Source: CAD feature listing. Evaluate the final solid. Frame: model axes, mm. A direction names the side the tool comes from. Round coordinates to 2 decimals unless told otherwise and drop trailing zeros. Loops run counter-clockwise (first coordinate to the right, second up) from the corner with the lowest first, then second, coordinate; pieces in that order, holes last. Notation, with made-up numbers: (-5.5, 79) - (32.5, 79) arc R16 cw to (32.5, 94) - close; hole circle Ø9 at (-39.5, 77.25). An arc over 180 degrees is marked (long way). One line per question, with ' | ' between items. Start each with the question number.
1. Mould query, pull axis Z, two halves, no side actions, for faces 4 (the flat face through (6.85, 18, -11)), 5 (the flat face through (-27.75, 14, 7)), 6 (the flat face through (0, 13, -11.75)), 7 (the flat face through (0, 13, 11.75)). Classes: pulls with the +Z half, pulls with the -Z half, needs draft (parallel to the pull), parting line crosses it, or undercut.
2. Ray query, line 1 (Z direction, x = 5.5, y = 4); line 2 (X direction, y = 15.25, z = 7.25); line 3 (Y direction, x = -4, z = 7.5). Return the intervals inside material, ascending.
3. Pin query (flat end, axial travel): pin 1 (1.5 mm diameter, centred on x = 18.5, z = 7.5, fed in from +Y); pin 2 (7 mm diameter, centred on x = -4.5, y = 17.5, fed in from -Z); pin 3 (1.5 mm diameter, centred on y = 18.5, z = 4.5, fed in from +X). Return the tip coordinate at first contact, or that it passes through.
4. Access query for faces 1 (the flat face through (-27.75, 14, -7)), 2 (the flat face through (0, 13.8, -11)), 3 (the flat face through (-29, 14, 5.75)). Directions: +Z, -Z, +X, -X, +Y, -Y. A direction counts if a zero-diameter tool reaches every point of the face in a straight line with its end or side. Return the directions, or none.
5. Cut plane D-D (x = 25.5). Return loops of the section in (y, z), then the cut area to 3 significant figures.
6. Cut plane A-A (y = 22). State how many separate pieces and enclosed holes the cut face has, then the cut area to 3 significant figures.
7. Cut plane B-B (x = 3). Return loops of the section in (y, z).
8. Cut plane C-C (y = 9). Return loops of the section in (x, z), then the cut area to 3 significant figures.
```python
from build123d import *

# Parameters (mm, degrees)
SKETCH1_W           = 61.5
SKETCH1_H           = 23.5
BOSS_EXTRUDE1_DEPTH = 3
BOSS_EXTRUDE2_DEPTH = 23
FILLET1_R           = 1
CUT_EXTRUDE1_REACH  = 48.624
FILLET2_R           = 1


with BuildPart() as part:
    # Sketch1 → Boss-Extrude1 (new body)
    with BuildSketch(Plane(origin=(0, 0, 0), x_dir=(1, 0, 0), z_dir=(0, 1, 0))):
        Rectangle(SKETCH1_W, SKETCH1_H)
    extrude(amount=BOSS_EXTRUDE1_DEPTH)

    # Sketch2 → Boss-Extrude2 (add)
    with BuildSketch(Plane(origin=(0, 3, 0), x_dir=(1, 0, 0), z_dir=(0, 1, 0))):
        Polygon((-27.75, -5.75), (-30.75, -5.75), (-30.75, -11.75), (30.75, -11.75), (30.75, -5.75), (27.75, -5.75), (27.75, -8.75), (-27.75, -8.75), align=None)
        Polygon((30.75, 5.75), (30.75, 11.75), (-30.75, 11.75), (-30.75, 5.75), (-27.75, 5.75), (-27.75, 8.75), (27.75, 8.75), (27.75, 5.75), align=None)
    extrude(amount=BOSS_EXTRUDE2_DEPTH)

    # Fillet1
    fillet1_edges = [part.edges().sort_by_distance(p)[0] for p in [
        (27.75, 14.5, 8.75),
        (-27.75, 14.5, 8.75),
        (-27.75, 14.5, -8.75),
        (27.75, 14.5, -8.75),
        (-30.75, 0, 0),
        (0, 0, 11.75),
        (30.75, 0, 0),
        (0, 0, -11.75),
        (-30.75, 13, -11.75),
        (-30.75, 13, 11.75),
        (30.75, 13, 11.75),
        (30.75, 13, -11.75),
    ]]
    fillet(fillet1_edges, radius=FILLET1_R)

    # Sketch3 → Cut-Extrude1 (cut, up to next)
    with BuildSketch(Plane(origin=(0, 0, -11.75), x_dir=(-1, 0, 0), z_dir=(0, 0, -1)), mode=Mode.PRIVATE) as cut_extrude1_sk1:
        Polygon((6.85, 13.8), (6.85, 23), (0, 23), (-6.85, 23), (-6.85, 13.8), align=None)
    cut_extrude1_tool1 = extrude(cut_extrude1_sk1.sketch, amount=-CUT_EXTRUDE1_REACH, mode=Mode.PRIVATE) & part.part
    add(cut_extrude1_tool1.solids().sort_by_distance((0, 18.4, -11.75))[0], mode=Mode.SUBTRACT)

    # Fillet2
    fillet2_edges = [part.edges().sort_by_distance(p)[0] for p in [
        (0, 23, -8.75),
        (-6.85, 18.4, -8.75),
        (0, 13.8, -8.75),
        (6.85, 18.4, -8.75),
    ]]
    fillet(fillet2_edges, radius=FILLET2_R)


solid = part.part
```
Answers follow:
1) face 4: needs draft | face 5: undercut | face 6: pulls with the -Z half | face 7: pulls with the +Z half
2) line 1: z = -11.75 to -8.75, 8.75 to 11.75 | line 2: x = -30.75 to -27.75, 27.75 to 30.75 | line 3: y = 0 to 3
3) pin 1: stops at y = 3 | pin 2: stops at z = -11.75 | pin 3: passes through
4) face 1: +Y | face 2: -Z | face 3: +X, -X, +Y
5) outline: (0, -10.75) arc R1 ccw to (1, -11.75) - (26, -11.75) - (26, -8.75) - (3, -8.75) - (3, 8.75) - (26, 8.75) - (26, 11.75) - (1, 11.75) arc R1 ccw to (0, 10.75) - close | area: 208 mm2
6) separate pieces: 3 | enclosed holes: 0 | area: 363 mm2
7) outline: (0, -10.75) arc R1 ccw to (1, -11.75) - (13.8, -11.75) - (13.8, -9.75) arc R1 ccw to (12.8, -8.75) - (3, -8.75) - (3, 8.75) - (26, 8.75) - (26, 11.75) - (1, 11.75) arc R1 ccw to (0, 10.75) - close; (23, -11.75) - (26, -11.75) - (26, -8.75) - (24, -8.75) arc R1 ccw to (23, -9.75) - close
8) outline: (-30.75, -10.75) arc R1 ccw to (-29.75, -11.75) - (29.75, -11.75) arc R1 ccw to (30.75, -10.75) - (30.75, -5.75) - (27.75, -5.75) - (27.75, -7.75) arc R1 cw to (26.75, -8.75) - (-26.75, -8.75) arc R1 cw to (-27.75, -7.75) - (-27.75, -5.75) - (-30.75, -5.75) - close; (-30.75, 5.75) - (-27.75, 5.75) - (-27.75, 7.75) arc R1 cw to (-26.75, 8.75) - (26.75, 8.75) arc R1 cw to (27.75, 7.75) - (27.75, 5.75) - (30.75, 5.75) - (30.75, 10.75) arc R1 ccw to (29.75, 11.75) - (-29.75, 11.75) arc R1 ccw to (-30.75, 10.75) - close | area: 405 mm2
